Could you check a few things on this model? Use its own coordinates, in mm. A direction names the side the tool comes from. Give positions to 0.01 mm unless a question says otherwise; leave off trailing zeros. Loops run counter-clockwise (first coordinate to the right, second up) from the corner with the lowest first, then second, coordinate; pieces in that order, holes last. Notation, with made-up numbers: M 15.25,-3.5 L 72.25,-3.5 A10 cw 72.25,5.5 Z; hole C 46.5,55.5 d11. An arc over 180 degrees is marked long. Use a Markdown table: item, result. Add a question column.
1) Which directions (+Z, -Z, +X, -X, +Y, -Y) give clear straight access to the entire face, cutting with the end or side of a thin tool? Please do faces 5 (the flat face through (6.96, 1.23, 2.97)), 6 (the cylindrical face through (9.4, 6.93, -3.17)), 7 (the cylindrical face through (2.335, 7.496, -14.93)), 8 (the cylindrical face through (-4.43, 3.73, 4.4)), 9 (the flat face through (8, 4, -10)).
2) If I drill on line 1 along X through (y, z) = (2.75, 0); line 2 along X through (y, z) = (2.1, 3); line 3 along Y through (x, z) = (9.5, 2.25), over which ranges is the centre line in solid material (lowest first)? Write a range as [from, to].
3) Will these pins go through, and if not, where does the flat tip stop? pin 1 Ø0.8 at (y, z) = (1, 3.5) entering from +X; pin 2 Ø0.8 at (y, z) = (6.5, 3) entering from +X; pin 3 Ø1 at (x, z) = (6, -14.5) entering from -Y; pin 4 Ø4.5 at (x, z) = (0, 0) entering from -Y.
4) Suppose I cut it at B-B on z = -8.5. List the corners of the cut face in (x, y) for me, and give its area (3 significant figures).
5) Suppose I cut it at A-A on z = 0. List the corners of the cut face in (x, y) for me.
6) We'd pull the mould along X, two halves only. Please class faces 1 (the flat face through (5, 7, 3)), 2 (the cylindrical face through (8.03, 3.79, 2.25)), 3 (the flat face through (-3, 4, -10)), 4 (the cylindrical face through (-4.43, 0.6, -3.59)): +X half, -X half, draft (parallel to the pull), parting line (faces both ways), or undercut.
7) Suppose I cut it at D-D on x = 1. List the corners of the cut face in (y, z) for me.
8) Suppose I cut it at C-C on y = 3.75. List the corners of the cut face in (x, z) for me, and give its area (3 significant figures).
```python
from build123d import *

# Parameters (mm, degrees)
SKETCH1_W           = 15
SKETCH1_H           = 15
SKETCH1_R           = 2.5
BOSS_EXTRUDE1_DEPTH = 7.5
SKETCH2_R           = 3.75
BOSS_EXTRUDE2_DEPTH = 10
SKETCH3_R           = 0.75
CUT_EXTRUDE1_DEPTH  = 7.5
CUT_EXTRUDE2_DEPTH  = 5
FILLET1_R           = 2


with BuildPart() as part:
    # Sketch1 → Boss-Extrude1 (new body)
    with BuildSketch(Plane(origin=(0, 0, 0), x_dir=(1, 0, 0), z_dir=(0, 1, 0))):
        with Locations((2.5, 2.5)):
            Rectangle(SKETCH1_W, SKETCH1_H)
        with Locations(Location((0, 0, 0), (0, 0, 270))):
            Circle(SKETCH1_R, mode=Mode.SUBTRACT)
    extrude(amount=BOSS_EXTRUDE1_DEPTH)

    # Sketch2 → Boss-Extrude2 (add)
    with BuildSketch(Plane(origin=(0, 0, -10), x_dir=(-1, 0, 0), z_dir=(0, 0, -1))):
        with Locations(Location((-2.5, 3.75, 0), (0, 0, 270))):
            Circle(SKETCH2_R)
    extrude(amount=BOSS_EXTRUDE2_DEPTH)

    # Sketch3 → Cut-Extrude1 (cut)
    with BuildSketch(Plane(origin=(0, 7.5, 0), x_dir=(1, 0, 0), z_dir=(0, 1, 0))):
        with Locations(Location((8, -3, 0), (0, 0, 270))):
            Circle(SKETCH3_R)
    extrude(amount=-CUT_EXTRUDE1_DEPTH, mode=Mode.SUBTRACT)

    # Sketch4 → Cut-Extrude2 (cut)
    with BuildSketch(Plane(origin=(10, 0, 0), x_dir=(0, 0, -1), z_dir=(1, 0, 0))):
        Polygon((-5, 7.5), (-1, 7.5), (-5, 5), align=None)
        Polygon((-5, 0), (-1, 0), (-5, 2.5), align=None)
    extrude(amount=-CUT_EXTRUDE2_DEPTH, mode=Mode.SUBTRACT)

    # Fillet1
    # the kernel refuses this fillet: 2 mm, written as the material it takes off along each edge
    with BuildSketch(Plane(origin=(-3, 2, 3), x_dir=(-1, 0, 0), z_dir=(0, 0, 1))) as fillet1_piece_1_section:
        Polygon((0, 0), (FILLET1_R, 0), (FILLET1_R, FILLET1_R), (0, FILLET1_R), align=None)
    fillet1_piece_1 = extrude(amount=FILLET1_R, mode=Mode.PRIVATE)
    fillet1_piece_1 = fillet1_piece_1 - Plane(origin=(-3, 2, 3), x_dir=(0.7071067811865475, 0.7071067811865475, 0), z_dir=(0, 0, 1)) * Sphere(FILLET1_R, mode=Mode.PRIVATE)
    add(fillet1_piece_1, mode=Mode.SUBTRACT)
    with BuildSketch(Plane(origin=(-3, 5.5, 3), x_dir=(-1, 0, 0), z_dir=(0, 0, 1))) as fillet1_piece_2_section:
        Polygon((0, 0), (FILLET1_R, 0), (FILLET1_R, -FILLET1_R), (0, -FILLET1_R), align=None)
    fillet1_piece_2 = extrude(amount=FILLET1_R, mode=Mode.PRIVATE)
    fillet1_piece_2 = fillet1_piece_2 - Plane(origin=(-3, 5.5, 3), x_dir=(0.7071067811865475, -0.7071067811865475, 0), z_dir=(0, 0, 1)) * Sphere(FILLET1_R, mode=Mode.PRIVATE)
    add(fillet1_piece_2, mode=Mode.SUBTRACT)
    with BuildSketch(Plane(origin=(10, -2.5, 5), x_dir=(-1, 0, 0), z_dir=(0, 1, 0))) as fillet1_piece_3:
        with BuildLine():
            CenterArc((FILLET1_R, -FILLET1_R), FILLET1_R, 90, 90)
            Line((0, -FILLET1_R), (0, 0))
            Line((0, 0), (FILLET1_R, 0))
        make_face()
    extrude(amount=12.5, mode=Mode.SUBTRACT)
    with BuildSketch(Plane(origin=(-5, 2, 5), x_dir=(1, 0, 0), z_dir=(0, 1, 0))) as fillet1_piece_4:
        with BuildLine():
            CenterArc((FILLET1_R, FILLET1_R), FILLET1_R, 180, 90)
            Line((0, FILLET1_R), (0, 0))
            Line((0, 0), (FILLET1_R, 0))
        make_face()
    extrude(amount=3.5, mode=Mode.SUBTRACT)
    with BuildSketch(Plane(origin=(-5, 0, -15), x_dir=(1, 0, 0), z_dir=(0, 0, 1))) as fillet1_piece_5:
        with BuildLine():
            CenterArc((FILLET1_R, FILLET1_R), FILLET1_R, 180, 90)
            Line((0, FILLET1_R), (0, 0))
            Line((0, 0), (FILLET1_R, 0))
        make_face()
    extrude(amount=18, mode=Mode.SUBTRACT)
    with BuildSketch(Plane(origin=(-5, 7.5, -15), x_dir=(1, 0, 0), z_dir=(0, 0, 1))) as fillet1_piece_6:
        with BuildLine():
            CenterArc((FILLET1_R, -FILLET1_R), FILLET1_R, 90, 90)
            Line((0, -FILLET1_R), (0, 0))
            Line((0, 0), (FILLET1_R, 0))
        make_face()
    extrude(amount=18, mode=Mode.SUBTRACT)
    with BuildSketch(Plane(origin=(-3, 0, 5), x_dir=(0, 1, 0), z_dir=(1, 0, 0))) as fillet1_piece_7:
        with BuildLine():
            CenterArc((FILLET1_R, -FILLET1_R), FILLET1_R, 90, 90)
            Line((0, -FILLET1_R), (0, 0))
            Line((0, 0), (FILLET1_R, 0))
        make_face()
    extrude(amount=13, mode=Mode.SUBTRACT)
    with BuildSketch(Plane(origin=(10, 0, 6), x_dir=(-1, 0, 0), z_dir=(0, 0, -1)), Plane(origin=(10, 7.5, 6), x_dir=(0, -1, 0), z_dir=(0, 0, -1))) as fillet1_piece_8:
        with BuildLine():
            CenterArc((FILLET1_R, FILLET1_R), FILLET1_R, 180, 90)
            Line((0, FILLET1_R), (0, 0))
            Line((0, 0), (FILLET1_R, 0))
        make_face()
    extrude(amount=21, mode=Mode.SUBTRACT)
    with BuildSketch(Plane(origin=(-3, 7.5, 5), x_dir=(0, -1, 0), z_dir=(1, 0, 0))) as fillet1_piece_9:
        with BuildLine():
            CenterArc((FILLET1_R, FILLET1_R), FILLET1_R, 180, 90)
            Line((0, FILLET1_R), (0, 0))
            Line((0, 0), (FILLET1_R, 0))
        make_face()
    extrude(amount=13, mode=Mode.SUBTRACT)


solid = part.part
```
Answer block:
| question | item | result |
|---|---|---|
| 1 | face 5 | +Z, +X, -Y |
| 1 | face 6 | +Z, -Z, +X, +Y |
| 1 | face 7 | -Z |
| 1 | face 8 | +Z, -X, +Y, -Y |
| 1 | face 9 | -Z, +X |
| 2 | line 1 | x = [-5, -2.5], [2.5, 10] |
| 2 | line 2 | x = [-5, 7.25], [8.75, 10] |
| 2 | line 3 | y = [0.78, 6.72] |
| 3 | pin 1 | stops at x = 5 |
| 3 | pin 2 | stops at x = 9.91 |
| 3 | pin 3 | stops at y = 1.5 |
| 3 | pin 4 | passes through |
| 4 | outline | M -5,2 A2 ccw -3,0 L 8,0 A2 ccw 10,2 L 10,5.5 A2 ccw 8,7.5 L -3,7.5 A2 ccw -5,5.5 Z |
| 4 | area | 109 mm^2 |
| 5 | outline | M -5,2 A2 ccw -3,0 L -2.5,0 L -2.5,7.5 L -3,7.5 A2 ccw -5,5.5 Z; M 2.5,0 L 8,0 A2 ccw 10,2 L 10,5.5 A2 ccw 8,7.5 L 2.5,7.5 Z |
| 6 | face 1 | +X half |
| 6 | face 2 | undercut |
| 6 | face 3 | draft |
| 6 | face 4 | -X half |
| 7 | outline | M 0,-10 L 0.31,-10 L 0.31,-20 L 7.19,-20 L 7.19,-10 L 7.5,-10 L 7.5,-2.29 L 0,-2.29 Z; M 0,2.29 L 7.5,2.29 L 7.5,3 A2 ccw 5.5,5 L 2,5 A2 ccw 0,3 Z |
| 8 | outline | M -5,-10 L -1.25,-10 L -1.25,-20 L 6.25,-20 L 6.25,-10 L 10,-10 L 10,3 A2 ccw 8,5 L -3,5 A2 ccw -5,3 Z; hole C 0,0 d5; hole C 8,3 d1.5 |
| 8 | area | 277 mm^2 |
